Design review of the part built by this model. Coordinates are the model's own, in mm. Coordinates: 2 decimals unless noted, no trailing zeros. Order: outer loops, then holes, each group sorted by start corner. A loop starts at its lowest first (then second) coordinate and runs counter-clockwise, first axis right, second up.
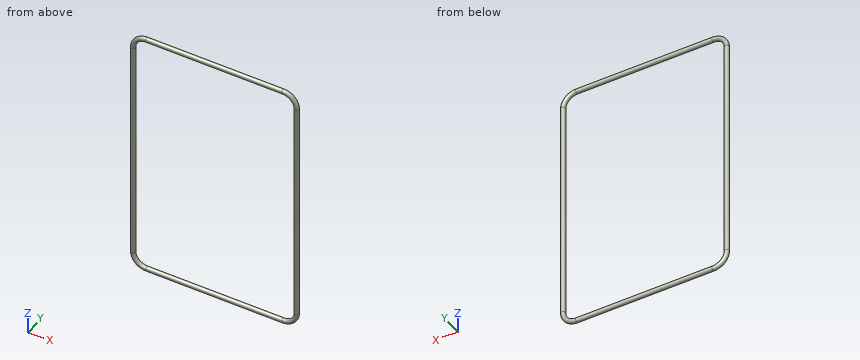
Autodesk Inventor part; units mm, degrees
ref_plane "YZ Plane" through (0, 0, 0) normal (1, 0, 0) x (0, 1, 0)
ref_plane "XZ Plane" through (0, 0, 0) normal (0, 1, 0) x (-1, 0, 0)
ref_plane "XY Plane" through (0, 0, 0) normal (0, 0, 1) x (1, 0, 0)
sketch "Sketch2" plane through (0, 0, 0) normal (0, 0, 1) x (1, 0, 0)
  circle A0 centre (0, 0) radius 0.7937
  dimension "d0" = 1.5875
sketch "Sketch3" plane through (0, 0, 0) normal (0, 1, 0) x (-1, 0, 0)
  line L0 (4.7625, 4.7625) -> (52.07, 4.7625)
  line L1 (56.8325, 0) -> (56.8325, -79.6925)
  line L2 (52.07, -84.455) -> (4.7625, -84.455)
  line L3 (0, -79.6925) -> (0, 0)
  arc A0 (56.8325, 0) -> (52.07, 4.7625) centre (52.07, 0) ccw
  arc A1 (52.07, -84.455) -> (56.8325, -79.6925) centre (52.07, -79.6925) ccw
  arc A2 (0, -79.6925) -> (4.7625, -84.455) centre (4.7625, -79.6925) ccw
  arc A3 (4.7625, 4.7625) -> (0, 0) centre (4.7625, 0) ccw
  dimension "d1" = 4.7625
  dimension "d2" = 89.2175
  dimension "d3" = 56.8325
sweep "Sweep1" add profiles "Sketch2" path "Sketch3"
properties part number "BatteryCaseORing" material "Rubber, Silicone"
1. Add section A-A (y = 0). Give the boundary of the cut face in (x, z), and give its area (3 significant figures).
2. Add section B-B (x = -35). Give the boundary of the cut face in (y, z) (1 decimal).
3. To check wall thickness, follow line 1 (X direction, y = -0.15, z = -12.5); line 2 (X direction, y = -0.05, z = -78); line 3 (Z direction, x = -24, y = 0.1). State the ranges of each line that lie inside material, in increasing order.
4. Add section C-C (z = -73). Give the boundary of the cut face in (x, y), and give its area (3 significant figures).
Solution:
1. outline: (-57.63, -79.69) arc R5.56 ccw to (-52.07, -85.25) - (-4.76, -85.25) arc R5.56 ccw to (0.79, -79.69) - (0.79, 0) arc R5.56 ccw to (-4.76, 5.56) - (-52.07, 5.56) arc R5.56 ccw to (-57.63, 0) - close; hole (-56.04, -79.69) arc R3.97 ccw to (-52.07, -83.66) - (-4.76, -83.66) arc R3.97 ccw to (-0.79, -79.69) - (-0.79, 0) arc R3.97 ccw to (-4.76, 3.97) - (-52.07, 3.97) arc R3.97 ccw to (-56.04, 0) - close
1. area: 451 mm2
2. outline: circle Ø1.6 at (0, -84.5); circle Ø1.6 at (0, 4.8)
3. line 1: x = -57.61 to -56.05, -0.78 to 0.78
3. line 2: x = -57.62 to -56.04, -0.79 to 0.79
3. line 3: z = -85.24 to -83.67, 3.98 to 5.55
4. outline: circle Ø1.59 at (-56.83, 0); circle Ø1.59 at (0, 0)
4. area: 3.96 mm2
